Autodesk Inventor part; units mm, degrees
ref_plane "YZ Plane" through (0, 0, 0) normal (1, 0, 0) x (0, 1, 0)
ref_plane "XZ Plane" through (0, 0, 0) normal (0, 1, 0) x (-1, 0, 0)
ref_plane "XY Plane" through (0, 0, 0) normal (0, 0, 1) x (1, 0, 0)
sketch "Sketch1" plane through (0, 0, 0) normal (0, 1, 0) x (-1, 0, 0)
  line L0 (5.4006, 7.1261) -> (-5.8039, 7.1261)
  line L1 (-5.8039, 7.1261) -> (-5.8039, -8.6499)
  line L2 (-5.8039, -8.6499) -> (5.4006, -8.6499)
  line L3 (5.4006, -8.6499) -> (5.4006, 7.1261)
  point P0 (0, 0)
extrude "Extrusion1" add sketch "Sketch1" along normal blind 5
sketch "Sketch2" plane through (5.8039, 0, 7.1261) normal (1, 0, 0) x (0, 0, -1)
  line L0 (0, 5) -> (15.7759, 5)
  circle A0 centre (5, 2.5) radius 2
  line L1 (0, 0) -> (0, 5)
  point P0 (7.1261, 0)
  dimension "d6" = 4
  dimension "d7" = 5
extrude "Extrusion2" cut sketch "Sketch2" against normal through all
fillet "Fillet1" radius 2 8 edges at (0.2017, 5, 7.1261) (0.2017, 0, 7.1261) (-5.4006, 5, -0.7619) (0.2017, 5, -8.6499) (0.2017, 0, -8.6499) (5.8039, 0, -0.7619) (5.8039, 5, -0.7619) (-5.4006, 0, -0.7619)
sketch "Sketch3" plane through (0, 5, 0) normal (0, 1, 0) x (1, 0, 0)
  circle A0 centre (0, 4.7093) radius 1.25
  point P0 (0, 0)
  dimension "d9" = 2.5
extrude "Extrusion3" cut sketch "Sketch3" against normal through all
properties part number "hands"
Could you check a few things on this model? Use its own coordinates, in mm. Round coordinates to 2 decimals unless told otherwise and drop trailing zeros. Loops run counter-clockwise (first coordinate to the right, second up) from the corner with the lowest first, then second, coordinate; pieces in that order, holes last. Notation, with made-up numbers: (56.25, 78) - (62.25, 78) arc R19 cw to (62.25, 84) - close; hole circle Ø4 at (-16.5, -4). An arc over 180 degrees is marked (long way). Answer in a Markdown table with one row per item. Add a question column.
(1) If we mould it in two halves opening along Y, with no side actions, what happens to faces 1 (the face through (0.28, 1.73, 0.28)), 2 (the face through (-4.83, 4.4, -0.87)), 3 (the face through (5.2, 0.57, -0.65))? For each: pulls with the +Y half, pulls with the -Y half, needs draft (parallel to the pull), parting line crosses it, or undercut.
(2) If we section it at B-B (y = 4): Please give me the cut outline in (x, z), plus the area to 3 significant figures.
(3) I need wall thicknesses on line 1 along Z through (x, y) = (0, 2.35); line 2 along Z through (x, y) = (-0.5, 0.85); line 3 along Z through (x, y) = (-3, 2.5). Which ranges of each line are inside material? Lowest first, please.
(4) If we section it at C-C (x = -2.75): Please give me the cut outline in (y, z).
(5) If we section it at D-D (z = -4): Please give me the cut outline in (x, y), plus the area to 3 significant figures.
(6) I'm going to push a flat-ended pin straight in: pin 1 (2.5 mm diameter, centred on y = 2.5, z = 2.13, fed in from +X). Where does the tip first touch, or does it pass through?
(7) If we section it at A-A (x = 0): Please give me the cut outline in (y, z).
Model answer:
| question | item | result |
|---|---|---|
| 1 | face 1 | undercut |
| 1 | face 2 | pulls with the +Y half |
| 1 | face 3 | pulls with the -Y half |
| 2 | outline | (-5.13, -8.38) - (5.54, -8.38) - (5.54, 0.8) - (-5.13, 0.8) - close; (-5.13, 3.45) - (5.54, 3.45) - (5.54, 6.86) - (-5.13, 6.86) - close; hole circle Ø2.5 at (0, -4.71) |
| 2 | area | 129 mm² |
| 3 | line 1 | z = -8.65 to -5.96, -3.46 to 0.13, 4.12 to 7.13 |
| 3 | line 2 | z = -8.29 to -5.85, -3.56 to 1, 3.26 to 6.76 |
| 3 | line 3 | z = -8.65 to 0.13, 4.13 to 7.13 |
| 4 | outline | (0, -6.65) arc R2 ccw to (2, -8.65) - (3, -8.65) arc R2 ccw to (5, -6.65) - (5, 5.13) arc R2 ccw to (3, 7.13) - (2, 7.13) arc R2 ccw to (0, 5.13) - close; hole circle Ø4 at (2.5, 2.13) |
| 5 | outline | (-5.4, 2) arc R2 ccw to (-3.4, 0) - (-1.03, 0) - (-1.03, 5) - (-3.4, 5) arc R2 ccw to (-5.4, 3) - close; (1.03, 0) - (3.8, 0) arc R2 ccw to (5.8, 2) - (5.8, 3) arc R2 ccw to (3.8, 5) - (1.03, 5) - close |
| 5 | area | 42.3 mm² |
| 6 | pin 1 | passes through |
| 7 | outline | (0, -6.65) arc R2 ccw to (2, -8.65) - (3, -8.65) arc R2 ccw to (5, -6.65) - (5, -5.96) - (0, -5.96) - close; (0, -3.46) - (5, -3.46) - (5, 5.13) arc R2 ccw to (3, 7.13) - (2, 7.13) arc R2 ccw to (0, 5.13) - close; hole circle Ø4 at (2.5, 2.13) |
